Source: CAD feature listing. Evaluate the final solid. Frame: model axes, mm. Face numbers are marked on the shaded views. Give positions to 0.01 mm unless a question says otherwise; leave off trailing zeros. Write each loop counter-clockwise with the first axis right and the second up, starting at its lowest first coordinate (ties: lowest second). Pieces come first, ordered by that corner, then holes. Notation, with made-up numbers: M -10,-24.75 L 27,-24.75 A14 ccw 27,-18.75 Z; hole C -22,-15 d4. An arc over 180 degrees is marked long. Return JSON: item names as keys, results as strings.
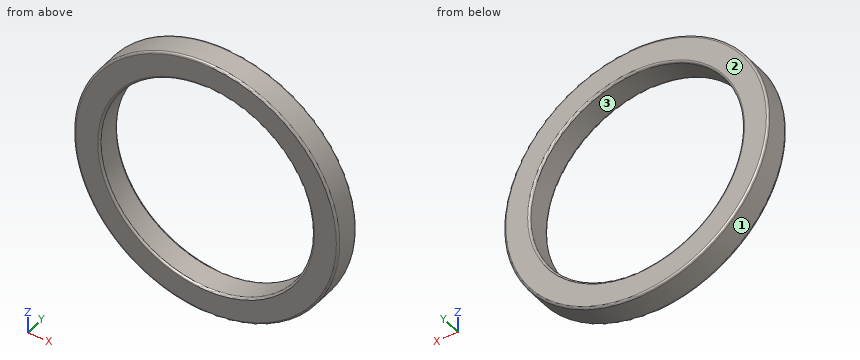
```python
from build123d import *

# Parameters (mm, degrees)
ESQUISSE1_W = 1.28
ESQUISSE1_H = 1.3
CONG_1_R    = 0.1


with BuildPart() as part:
    # Esquisse1 → Révolution1 (revolve)
    with BuildSketch(Plane.XY):
        with Locations((5.91, 2.321727173)):
            Rectangle(ESQUISSE1_W, ESQUISSE1_H)
    revolve(axis=Axis((0, 0, 0), (0, 1, 0)))

    # Congé1
    cong_1_edges = [part.edges().sort_by_distance(p)[0] for p in [
        (-5.27, 2.971727173, 0),
        (-6.55, 2.971727173, 0),
        (-6.55, 1.671727173, 0),
        (-5.27, 1.671727173, 0),
    ]]
    fillet(cong_1_edges, radius=CONG_1_R)


solid = part.part
```
1) Draft query along X for the marked faces 1, 2 and 3. Return one class per face: released by +X, released by -X, zero draft, split by the parting line, or undercut.
Numbers:
{"face 1": "split by the parting line", "face 2": "zero draft", "face 3": "undercut"}
2) Line query: line 1 (X direction, y = 2.05, z = 0); line 2 (X direction, y = 1.95, z = 0.5). Output: solid intervals per line, ascending. Write a range as [from, to].
Numbers:
{"line 1": "x = [-6.55, -5.27], [5.27, 6.55]", "line 2": "x = [-6.53, -5.25], [5.25, 6.53]"}
3) Cut plane A-A, the plane z = 0. Return the cut outline in (x, y), then the cut area to 3 significant figures.
Numbers:
{"outline": "M -6.55,1.77 A0.1 ccw -6.45,1.67 L -5.37,1.67 A0.1 ccw -5.27,1.77 L -5.27,2.87 A0.1 ccw -5.37,2.97 L -6.45,2.97 A0.1 ccw -6.55,2.87 Z; M 5.27,1.77 A0.1 ccw 5.37,1.67 L 6.45,1.67 A0.1 ccw 6.55,1.77 L 6.55,2.87 A0.1 ccw 6.45,2.97 L 5.37,2.97 A0.1 ccw 5.27,2.87 Z", "area": "3.31 mm²"}
4) Cut plane B-B, the plane x = 0. Return the cut outline in (y, z), then the cut area to 3 significant figures.
Numbers:
{"outline": "M 1.67,-6.45 A0.1 ccw 1.77,-6.55 L 2.87,-6.55 A0.1 ccw 2.97,-6.45 L 2.97,-5.37 A0.1 ccw 2.87,-5.27 L 1.77,-5.27 A0.1 ccw 1.67,-5.37 Z; M 1.67,5.37 A0.1 ccw 1.77,5.27 L 2.87,5.27 A0.1 ccw 2.97,5.37 L 2.97,6.45 A0.1 ccw 2.87,6.55 L 1.77,6.55 A0.1 ccw 1.67,6.45 Z", "area": "3.31 mm²"}
5) Cut plane C-C, the plane y = 2.7. Return the cut outline in (x, z).
Numbers:
{"outline": "C 0,0 d13.1; hole C 0,0 d10.54"}
